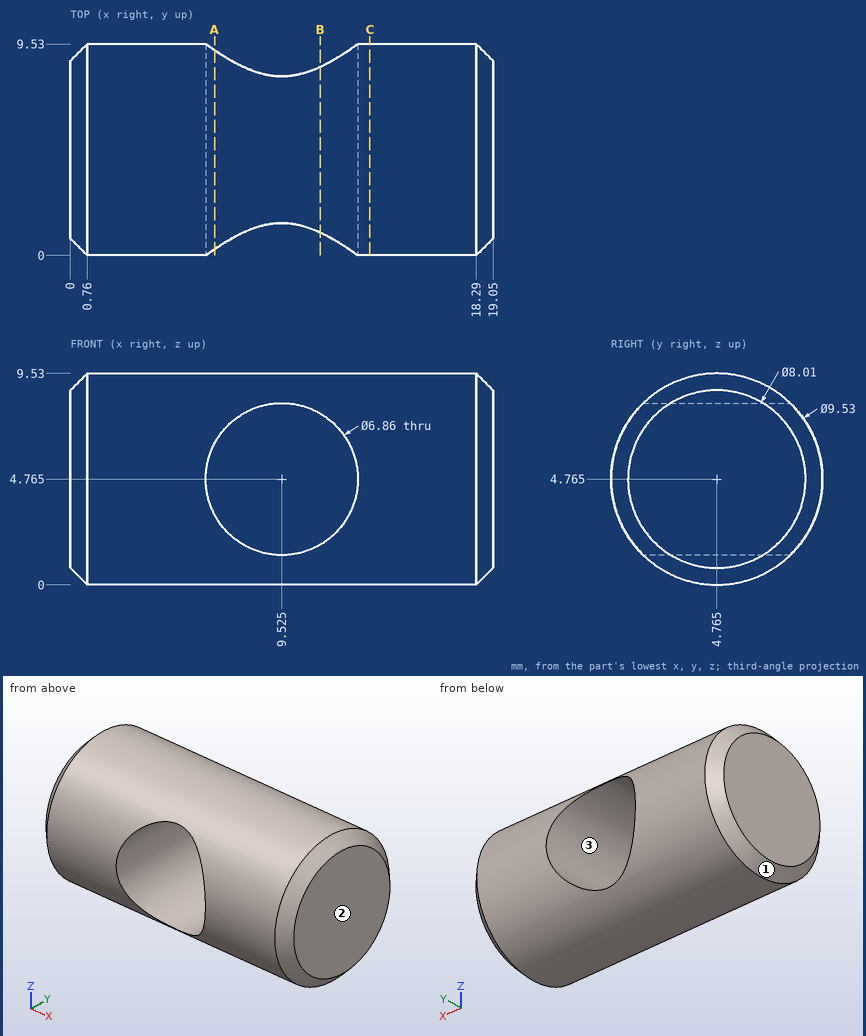
Geometry: see drawing. Coordinates: mm, zero at the bounding-box minimum. Round coordinates to 2 decimals unless told otherwise and drop trailing zeros. Write each loop counter-clockwise with the first axis right and the second up, starting at its lowest first coordinate (ties: lowest second). Pieces come first, ordered by that corner, then holes. Notation, with made-up numbers: (-23, 59.25) -> (-11, 59.25) arc R25 cw to (-11, 85.25) -> close; hole circle Ø10 at (16, 38.25). An arc over 180 degrees is marked (long way). Answer as CSV lines item,"result".
1. Contact query for flat-ended pins moving along their axis: P1, Ø2, axis at x = 13, z = 6.5, coming from the +Y side; P2, Ø5, axis at x = 16.5, y = 7.5, coming from the +Z side; P3, Ø3, axis at x = 10.5, z = 1, coming from the -Y side. Output: stop coordinate, or through.
Geometry says:
P1,"stops at y = 9.47"
P2,"stops at z = 9.52"
P3,"stops at y = 0.86"
2. Section A-A (x = 6.5). Return the cut outline in (y, z) (3 decimals).
Geometry says:
outline,"(0.283, 3.148) arc R4.765 ccw to (9.247, 3.148) -> close; (0.283, 6.382) -> (9.247, 6.382) arc R4.765 ccw to start"
3. Mould query, pull axis Z, two halves, no side actions, for the marked faces 1, 2 and 3. Classes: +Z half, -Z half, draft (parallel to the pull), parting line (faces both ways), or undercut.
Geometry says:
face 1,"parting line"
face 2,"draft"
face 3,"undercut"
4. Section B-B (x = 11.25). Return the cut outline in (y, z) (3 decimals), plus the area to 3 significant figures.
Geometry says:
outline,"(1.035, 1.8) arc R4.765 ccw to (8.495, 1.8) -> close; (1.035, 7.73) -> (8.495, 7.73) arc R4.765 ccw to start"
area,"18.7 mm^2"
5. Section C-C (x = 13.5). Return the cut outline in (y, z) (3 decimals).
Geometry says:
outline,"circle Ø9.53 at (4.765, 4.765)"
6. Ray query, L1, parallel to X at y = 1.5, z = 1.75; L2, parallel to X at y = 1.25, z = 7.5; L3, parallel to Z at x = 11.75, y = 4.75. Return the intervals inside material, ascending. Write a range as [from, to].
Geometry says:
L1,"x = [0.44, 7.89], [11.16, 18.61]"
L2,"x = [0.45, 7.46], [11.59, 18.6]"
L3,"z = [0, 2.15], [7.38, 9.53]"
